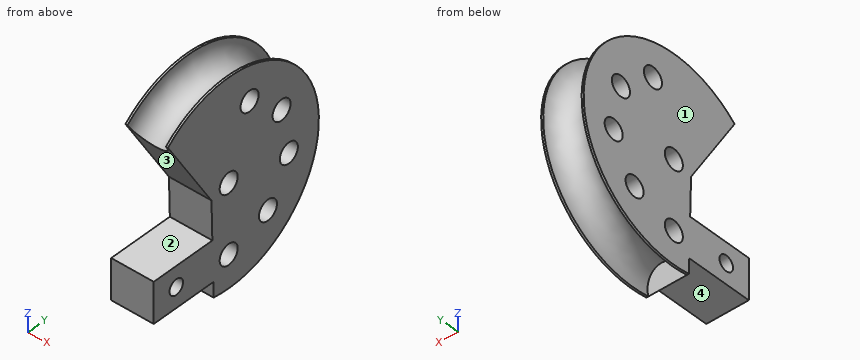
from build123d import *

# Parameters (mm, degrees)
F0_R     = 9.525
F0_R_2   = 12.7
F1_DEPTH = 53.34


with BuildPart() as f1:
    # F0 (on Right) → F1 (new body)
    with BuildSketch(Plane.YZ):
        with BuildLine():
            Line((-21.7306433309, -106.1653788452), (-21.2513333333, -125.2093480198))
            ThreePointArc((-21.2513333333, -125.2093480198), (121.8537281077, 35.7864352271), (-85.5809014362, 93.8344782549))
            Line((-85.5809014362, 93.8344782549), (-24.2392100937, -6.4948767698))
            Line((-24.2392100937, -6.4948767698), (-23.0092080907, -55.3653788452))
            Line((-23.0092080907, -55.3653788452), (-105.5592080907, -55.3653788452))
            Line((-105.5592080907, -55.3653788452), (-105.5592080907, -106.1653788452))
            Line((-105.5592080907, -106.1653788452), (-21.7306433309, -106.1653788452))
        make_face()
        with Locations((-73.8092080907, -80.7653788452)):
            Circle(F0_R, mode=Mode.SUBTRACT)
        with Locations((0, -86.0425)):
            Circle(F0_R_2, mode=Mode.SUBTRACT)
        with Locations((55.3070529065, -65.9123789971)):
            Circle(F0_R_2, mode=Mode.SUBTRACT)
        with Locations((84.7353210886, -14.9411233269)):
            Circle(F0_R_2, mode=Mode.SUBTRACT)
        Circle(F0_R_2, mode=Mode.SUBTRACT)
        with Locations((74.5149908051, 43.02125)):
            Circle(F0_R_2, mode=Mode.SUBTRACT)
        with Locations((29.4282681821, 80.853502324)):
            Circle(F0_R_2, mode=Mode.SUBTRACT)
    extrude(amount=F1_DEPTH)

    # F3: sweep along a path in F3_path
    with BuildLine(Plane(origin=(53.34, -21.2513333333, -125.2093480198), x_dir=(0, 0, 1), z_dir=(1, 0, 0))) as f3_path:
        ThreePointArc((0, 0), (160.995783247, -143.105061441), (219.0438262748, 64.3295681028))
    # F2 (on face) → F3 (sweep, cut)
    with BuildSketch(Plane(origin=(0, -20.5342212669, -12.5546891296), x_dir=(1, 0, 0), z_dir=(0, -0.8531709236, -0.5216314552))):
        with BuildLine():
            ThreePointArc((2.54, 124.6985386355), (26.67, 100.5685386355), (50.8, 124.6985386355))
            Line((50.8, 124.6985386355), (2.54, 124.6985386355))
        make_face()
        with BuildLine():
            Line((2.54, 124.6985386355), (50.8, 124.6985386355))
            ThreePointArc((50.8, 124.6985386355), (26.67, 148.8285386355), (2.54, 124.6985386355))
        make_face()
    sweep(path=f3_path.line, mode=Mode.SUBTRACT)


solid = f1.part
Here's how the part is built. I have some questions about the finished solid (model axes, mm). Face numbers are marked on the shaded views. Give positions to 0.01 mm unless a question says otherwise; leave off trailing zeros. Write each loop counter-clockwise with the first axis right and the second up, starting at its lowest first coordinate (ties: lowest second). Pieces come first, ordered by that corner, then holes. Notation, with made-up numbers: (-38, 40.25) -> (18, 40.25) arc R22 cw to (18, 46.25) -> close; hole circle Ø2 at (23, 11). An arc over 180 degrees is marked (long way). Use one line per item in the form item = value. Start each with the question number.
1. Imagine slicing it at A-A on y = 0. State how many separate pieces and enclosed holes the cut face has, plus the area to 3 significant figures.
2. Imagine slicing it at B-B on y = -89.5. List the corners of the cut face in (x, z) for me.
3. If I drill on L1, parallel to Z at x = 22.5, y = 0; L2, parallel to Z at x = 30.5, y = -7; L3, parallel to Y at x = 19, z = -94.5, over which ranges is the centre line in solid material (lowest first)?
4. Thinking about a two-plate mould opening in Z: for the marked faces 1, 2, 3 and 4, which applies, +Z half, -Z half, draft (parallel to the pull), parting line (faces both ways), or undercut?
5. Will these pins go through, and if not, where does the flat tip stop? pin 1 Ø2 at (y, z) = (-59.5, 51) entering from +X; pin 2 Ø2 at (x, y) = (35.5, 22) entering from +Z; pin 3 Ø15 at (y, z) = (74.51, 43.02) entering from -X; pin 4 Ø6 at (x, y) = (11, 15) entering from -Z.
Entries:
q1.separate_pieces = 3
q1.enclosed_holes = 0
q1.area = 9,050 mm²
q2.outline = (0, -106.17) -> (53.34, -106.17) -> (53.34, -55.37) -> (0, -55.37) -> close
q3.L1 = -103.76 to -98.74, -73.34 to -12.7, 12.7 to 103.76
q3.L2 = -103.47 to -96.64, -75.45 to -10.6, 10.6 to 103.47
q3.L3 = -105.56 to -9.47, 9.47 to 44.9
q4.face_1 = draft
q4.face_2 = undercut
q4.face_3 = undercut
q4.face_4 = -Z half
q5.pin_1 = 53.34
q5.pin_2 = 103.17
q5.pin_3 = through
q5.pin_4 = -111.04
